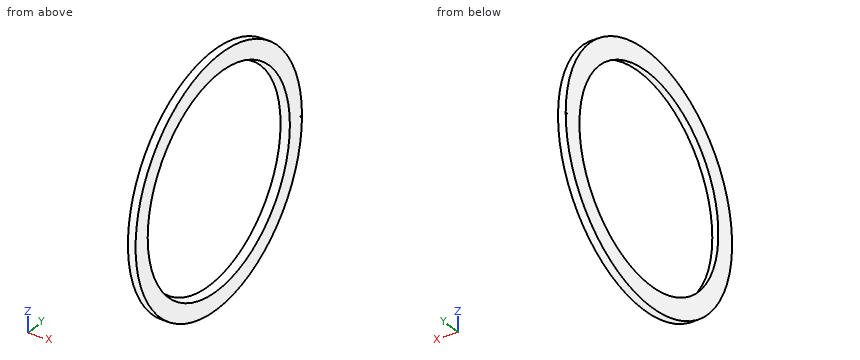
Autodesk Inventor part; units mm, degrees
ref_plane "YZ Plane" through (0, 0, 0) normal (1, 0, 0) x (0, 1, 0)
ref_plane "XZ Plane" through (0, 0, 0) normal (0, 1, 0) x (-1, 0, 0)
ref_plane "XY Plane" through (0, 0, 0) normal (0, 0, 1) x (1, 0, 0)
sketch "Sketch1" plane through (0, 0, 0) normal (0, 0, 1) x (1, 0, 0)
  arc A0 (180.1312, 23.4516) -> (181.5833, 23.6751) centre (180.1312, 28.2803) ccw
  arc A1 (180.1312, 23.4516) -> (181.5842, 23.6753) centre (180.1312, 28.2803) ccw
  arc A2 (167.724, 26.7761) -> (180.1312, 23.4516) centre (180.1312, 48.266) ccw
  arc A3 (166.724, 25.044) -> (180.1312, 21.4516) centre (180.1312, 48.266) ccw
  line L0 (125.6541, 47.7887) -> (168.987, 22.7705)
  line L1 (124.6541, 46.0566) -> (167.987, 21.0384)
  arc A4 (180.1312, 21.4516) -> (182.1847, 21.7676) centre (180.1312, 28.2803) ccw
  arc A5 (124.6541, 46.0566) -> (31.2848, 71.0749) centre (31.2848, -115.6637) ccw
  arc A6 (125.6541, 47.7887) -> (31.2848, 73.0749) centre (31.2848, -115.6637) ccw
  line L2 (1.263, 71.0749) -> (31.2848, 71.0749)
  line L3 (1.263, 73.0749) -> (31.2848, 73.0749)
  line L4 (236.5136, 40.9945) -> (181.5833, 23.6751)
  line L5 (182.1847, 21.7676) -> (237.115, 39.0871)
  line L6 (1.263, -0.4301) -> (320.4324, -0.4301)
  line L7 (236.5136, 40.9945) -> (237.115, 39.0871)
  line L8 (1.263, 84.1749) -> (31.2848, 84.1749)
  line L9 (167.987, 21.0384) -> (167.987, -8.65)
  line L10 (31.2848, 84.1749) -> (166.987, 84.1749)
  line L11 (233.5136, 47.8077) -> (145.7323, 20.1304)
  line L12 (234.2883, 48.052) -> (238.3779, 48.052)
  line L13 (234.2883, 48.052) -> (168.987, 48.052)
  line L14 (168.987, 86.1749) -> (31.2848, 86.1749)
  line L15 (31.2848, 86.1749) -> (1.263, 86.1749)
  line L16 (234.2883, 50.052) -> (170.987, 50.052)
  line L17 (169.987, 21.0384) -> (169.987, 27.7779)
  line L18 (169.987, 51.052) -> (169.987, 85.1749)
  line L19 (167.987, 21.0384) -> (167.987, 27.1473)
  line L20 (167.987, 49.052) -> (167.987, 83.1749)
  arc A7 (167.987, 83.1749) -> (166.987, 84.1749) centre (166.987, 83.1749) ccw
  arc A8 (169.987, 85.1749) -> (168.987, 86.1749) centre (168.987, 85.1749) ccw
  arc A9 (169.987, 51.052) -> (170.987, 50.052) centre (170.987, 51.052) ccw
  arc A10 (167.987, 49.052) -> (168.987, 48.052) centre (168.987, 49.052) ccw
  line L21 (1.263, 84.1749) -> (1.263, 86.1749)
  line L22 (238.3779, 48.052) -> (238.3779, 50.052)
  line L23 (234.2883, 50.052) -> (238.3779, 50.052)
  line L24 (236.5136, 40.9945) -> (236.5136, 48.052)
  line L25 (236.5136, 48.052) -> (233.5136, 48.052)
  line L26 (233.5136, 48.052) -> (233.5136, 40.0486)
  line L27 (233.5136, 48.052) -> (234.2883, 48.052)
  line L28 (233.5136, 48.052) -> (233.5136, 47.8077)
  dimension "d40" = 30.0219
  dimension "d41" = 186.7386
  dimension "d42" = 0
  dimension "d43" = 0
  dimension "d44" = 71.505
  dimension "d45" = 2
  dimension "d46" = 2
  dimension "d47" = 2
  dimension "d48" = 2
  dimension "d49" = 2
  dimension "d50" = 17.5
  dimension "d51" = 54.9303
  dimension "d52" = 2
  dimension "d53" = 11.1
  dimension "d54" = 7.4
  dimension "d55" = 17.5
  dimension "d56" = 2
  dimension "d57" = 2
  dimension "d58" = 1
  dimension "d59" = 1
  dimension "d60" = 1
  dimension "d61" = 1
  dimension "d62" = 3
revolve "Revolution1" add sketch "Sketch1" angle 360 about axis through (1.263, -0.4301, 0) along (1, 0, 0) contours L26 L13 L12 L24 L4
sketch "Sketch2" plane through (236.5136, -0.4301, 0) normal (1, 0, 0) x (0, 0, -1)
  circle A0 centre (0, 0) radius 41.4246
  line L0 (0, 41.4246) -> (0, 46.1871)
  circle A1 centre (0, 46.1871) radius 4.7625
  point P0 (0, 0.4301)
  dimension "d63" = 4.7625
  dimension "d64" = 9.525
sketch "Sketch5" plane through (236.5136, -0.4301, 0) normal (1, 0, 0) x (0, 0, -1)
  circle A0 centre (0, 42.1815) radius 4.7625
  circle A1 centre (0, 0) radius 48.4822
  line L0 (0, 48.4822) -> (0, 47.9822)
  line L1 (0.25, 47.7322) -> (-0.25, 47.7322)
  line L2 (-0.25, 47.7322) -> (-0.25, 48.2322)
  line L3 (-0.25, 48.2322) -> (0.25, 48.2322)
  line L4 (0.25, 48.2322) -> (0.25, 47.7322)
  line L5 (0.25, 47.7322) -> (-0.25, 48.2322) construction
  line L6 (-0.25, 47.7322) -> (0.25, 48.2322) construction
  point P0 (0, 0.4301)
  point P1 (0, 41.4246)
  dimension "d72" = 0.5
  dimension "d76" = 0.5
  dimension "d77" = 0.5
extrude "Extrusion1" cut sketch "Sketch5" against normal blind 3.5 contours L3 L4 L1 L2
properties part number "back bracket" material "Stainless Steel"
The listing builds one solid part. Answer for the finished solid, in the listing's coordinates (mm). Coordinates: 2 decimals unless noted, no trailing zeros. Loops run counter-clockwise (first coordinate to the right, second up) from the corner with the lowest first, then second, coordinate; pieces in that order, holes last. Notation, with made-up numbers: (-21, 7.5) -> (29, 7.5) arc R16 ccw to (29, 29.5) -> close; hole circle Ø8 at (17, -16.75). An arc over 180 degrees is marked (long way). Return JSON: item names as keys, results as strings. Group by question number.
(1) A cutting plane is placed at A-A on x = 235.85. Write down the section's boundary in (y, z).
(2) Given pin 1 Ø1 at (x, z) = (235.5, -9) entering from -Y; pin 2 Ø1 at (x, y) = (236, 32) entering from -Z, each flat-ended and moving along its own axis, determine where each tip first touches the part or whether it passes through.
(3) Find the intervals of material crossed by probe 1 along Y at (x, z) = (236, 2.5); probe 2 along Z at (x, y) = (235.05, -3.5); probe 3 along Z at (x, y) = (233.9, 12), in increasing order. Write a range as from..to.
The answers:
{
 "1": {"outline": "circle Ø96.96 at (-0.43, 0); hole circle Ø82.43 at (-0.43, 0); hole (47.3, -0.25) -> (47.8, -0.25) -> (47.8, 0.25) -> (47.3, 0.25) -> close"},
 "2": {"pin 1": "stops at y = -48.16", "pin 2": "stops at z = -36.48"},
 "3": {"probe 1": "y = -48.85..-41.62, 40.76..47.99", "probe 2": "z = -48.38..-40.85, 40.85..48.38", "probe 3": "z = -46.86..-38.65, 38.65..46.86"}
}
